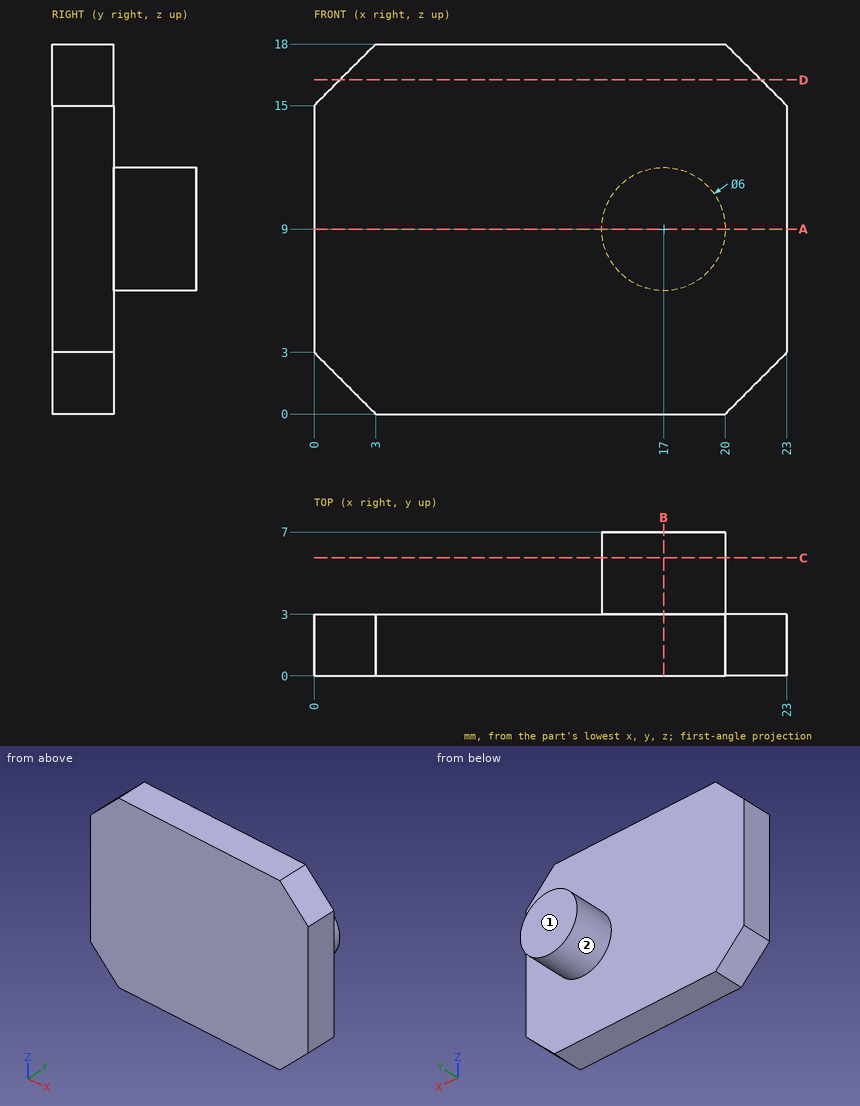
Job drawing, mm, ordinate dimensions from the low corner. One solid piece. A direction names the side the tool comes from. Coordinates: 2 decimals unless noted, no trailing zeros. Write each loop counter-clockwise with the first axis right and the second up, starting at its lowest first coordinate (ties: lowest second). Pieces come first, ordered by that corner, then holes. Notation, with made-up numbers: M -5,69.25 L 44,69.25 A19 ccw 44,79.25 Z; hole C -14,10 d10. An arc over 180 degrees is marked long. Answer as a JSON object with one key per item and string values. Group by question number.
1) Saw through at D-D (z = 16.25). Write the cut outline in (x, y), plus the area to 3 significant figures.
2) Saw through at A-A (z = 9). Write the cut outline in (x, y), plus the area to 3 significant figures.
3) Saw through at B-B (x = 17). Write the cut outline in (y, z).
4) Tool access for the marked faces 1 and 2: list every direction of +Z, -Z, +X, -X, +Y, -Y with a clear straight run to the whole face (end or side of a thin tool).
5) Pin check, flat tips, straight feed: pin 1 Ø3 at (x, y) = (20.5, 5) entering from -Z; pin 2 Ø3 at (x, z) = (5.5, 6) entering from +Y. Stop position of each tip, or through.
6) Wall check: line 1 (Y direction, x = 6.25, z = 13.75); line 2 (Z direction, x = 18, y = 6.5); line 3 (X direction, y = 5.5, z = 9). Give the ranges that are in metal, low to high. Write a range as from..to.
7) Saw through at C-C (y = 5.75). Write the cut outline in (x, z).
Values follow:
{
 "1": {"outline": "M 1.25,0 L 21.75,0 L 21.75,3 L 1.25,3 Z", "area": "61.5 mm2"},
 "2": {"outline": "M 0,0 L 23,0 L 23,3 L 20,3 L 20,7 L 14,7 L 14,3 L 0,3 Z", "area": "93.0 mm2"},
 "3": {"outline": "M 0,0 L 3,0 L 3,6 L 7,6 L 7,12 L 3,12 L 3,18 L 0,18 Z"},
 "4": {"face 1": "+Z, -Z, +X, -X, +Y", "face 2": "+Y"},
 "5": {"pin 1": "stops at z = 6.76", "pin 2": "stops at y = 3"},
 "6": {"line 1": "y = 0..3", "line 2": "z = 6.17..11.83", "line 3": "x = 14..20"},
 "7": {"outline": "C 17,9 d6"}
}
